Solid Edge part; units mm, degrees
sketch "Sketch1" plane through (0, 0, 0) normal (0, 0, 1) x (1, 0, 0)
  line L0 (-11.53, 6.55) -> (-11.53, -44.45)
  line L1 (-11.53, -44.45) -> (13.97, -44.45)
  line L2 (13.97, -44.45) -> (13.97, 6.55)
  line L3 (13.97, 6.55) -> (-11.53, 6.55)
extrude "Protrusion1" add sketch "Sketch1" along normal blind 1.5875
sketch "Sketch2" plane through (1.22, -18.95, 1.5875) normal (0, 0, 1) x (1, 0, 0)
  circle A0 centre (-10.375, 22.505) radius 1.55
  circle A1 centre (10.375, 22.505) radius 1.55
  circle A2 centre (10.375, -22.505) radius 1.55
  circle A3 centre (-10.375, -22.505) radius 1.55
extrude "ExtrudedCutout_1" cut sketch "Sketch2" against normal blind 58.166
For this review, take the finished solid that the model builds, in its own axes (mm). Round coordinates to 2 decimals unless told otherwise and drop trailing zeros. Write each loop counter-clockwise with the first axis right and the second up, starting at its lowest first coordinate (ties: lowest second). Pieces come first, ordered by that corner, then holes. Notation, with made-up numbers: (-34.5, -9) -> (18.5, -9) arc R27 cw to (18.5, 13) -> close; hole circle Ø3 at (12, 10.25). An arc over 180 degrees is marked (long way). Put each result on its own line as item: value.
Q1. Consider section B-B on x = -9. State the section outline as (y, z) points.
Determined:
outline: (-44.45, 0) -> (-43, 0) -> (-43, 1.59) -> (-44.45, 1.59) -> close; (-39.91, 0) -> (2.01, 0) -> (2.01, 1.59) -> (-39.91, 1.59) -> close; (5.1, 0) -> (6.55, 0) -> (6.55, 1.59) -> (5.1, 1.59) -> close
Q2. To check wall thickness, follow L1, parallel to Y at x = -8.5, z = 0.4; L2, parallel to Y at x = -8.75, z = 1.2. State the ranges of each line that lie inside material, in increasing order. Write a range as [from, to].
Determined:
L1: y = [-44.45, -42.86], [-40.05, 2.15], [4.96, 6.55]
L2: y = [-44.45, -42.95], [-39.96, 2.06], [5.05, 6.55]
Q3. Consider section A-A on z = 0.6. State the section outline as (x, y) points (3 decimals).
Determined:
outline: (-11.53, -44.45) -> (13.97, -44.45) -> (13.97, 6.55) -> (-11.53, 6.55) -> close; hole circle Ø3.1 at (-9.155, -41.455); hole circle Ø3.1 at (-9.155, 3.555); hole circle Ø3.1 at (11.595, -41.455); hole circle Ø3.1 at (11.595, 3.555)
Q4. Clearance check with a flat-ended pin moving along its axis: pin 1 Ø1.9 at (x, y) = (-9.155, -41.455) entering from +Z. State where the tip first meets the part, or that it passes through.
Determined:
pin 1: passes through
Q5. The part is to be moulded in two halves that separate along X. For faces 1 (the cylindrical face through (-10.385, 2.612, 0.805)), 2 (the flat face through (13.97, -19, 1)), 3 (the flat face through (1, -19, 1.588)), say which applies: released by +X, released by -X, zero draft, split by the parting line, or undercut.
Determined:
face 1: undercut
face 2: released by +X
face 3: zero draft
